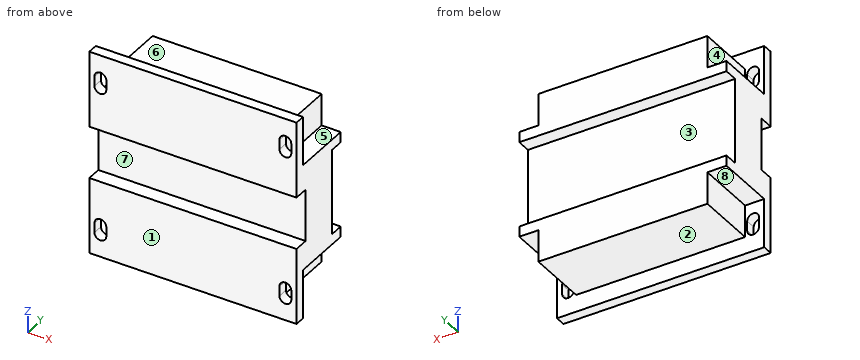
```python
from build123d import *

# Parameters (mm, degrees)
SKETCH1_W           = 75.692
SKETCH1_H           = 62.23
BOSS_EXTRUDE1_DEPTH = 25.908
SKETCH2_W           = 75.692
SKETCH2_H           = 31.242
CUT_EXTRUDE1_DEPTH  = 5.08
SKETCH4_W           = 6.985
SKETCH4_H           = 11.684
CUT_EXTRUDE4_DEPTH  = 22.098
SKETCH3_W           = 75.692
SKETCH3_H           = 19.05
CUT_EXTRUDE5_DEPTH  = 5.334
SKETCH8_W           = 75.692
SKETCH8_H           = 3.81
BOSS_EXTRUDE2_DEPTH = 6.223
SKETCH9_W           = 75.692
SKETCH9_H           = 3.81
BOSS_EXTRUDE3_DEPTH = 6.223
CUT_EXTRUDE6_REACH  = 84.92


with BuildPart() as part:
    # Sketch1 → Boss-Extrude1 (new body)
    with BuildSketch(Plane(origin=(0, 0, 0), x_dir=(1, 0, 0), z_dir=(0, 1, 0))):
        with Locations((-20.973907218, -15.051745981)):
            Rectangle(SKETCH1_W, SKETCH1_H)
    extrude(amount=BOSS_EXTRUDE1_DEPTH)

    # Sketch2 → Cut-Extrude1 (cut)
    with BuildSketch(Plane(origin=(0, 25.908, 0), x_dir=(1, 0, 0), z_dir=(0, 1, 0))):
        with Locations((-20.973907218, -15.051745981)):
            Rectangle(SKETCH2_W, SKETCH2_H)
    extrude(amount=-CUT_EXTRUDE1_DEPTH, mode=Mode.SUBTRACT)

    # Sketch4 → Cut-Extrude4 (cut)
    with BuildSketch(Plane(origin=(0, 25.908, 0), x_dir=(1, 0, 0), z_dir=(0, 1, 0))):
        with Locations((13.379592782, -40.324745981)):
            Rectangle(SKETCH4_W, SKETCH4_H)
        with Locations((-55.327407218, -40.324745981)):
            Rectangle(SKETCH4_W, SKETCH4_H)
        with Locations((-55.327407218, 10.221254019)):
            Rectangle(SKETCH4_W, SKETCH4_H)
        with Locations((13.379592782, 10.221254019)):
            Rectangle(SKETCH4_W, SKETCH4_H)
    extrude(amount=-CUT_EXTRUDE4_DEPTH, mode=Mode.SUBTRACT)

    # Sketch3 → Cut-Extrude5 (cut)
    with BuildSketch(Plane.XZ):
        with Locations((-20.973907218, 15.051745981)):
            Rectangle(SKETCH3_W, SKETCH3_H)
    extrude(amount=-CUT_EXTRUDE5_DEPTH, mode=Mode.SUBTRACT)

    # Sketch8 → Boss-Extrude2 (add)
    with BuildSketch(Plane.XY.offset(46.166745981)):
        with Locations((-20.973907218, 1.905)):
            Rectangle(SKETCH8_W, SKETCH8_H)
    extrude(amount=BOSS_EXTRUDE2_DEPTH)

    # Sketch9 → Boss-Extrude3 (add)
    with BuildSketch(Plane(origin=(0, 0, -16.063254019), x_dir=(-1, 0, 0), z_dir=(0, 0, -1))):
        with Locations((20.973907218, 1.905)):
            Rectangle(SKETCH9_W, SKETCH9_H)
    extrude(amount=BOSS_EXTRUDE3_DEPTH)

    # Sketch7 → Cut-Extrude6 (cut, up to next)
    with BuildSketch(Plane.XZ, mode=Mode.PRIVATE) as cut_extrude6_sk1:
        with BuildLine():
            Line((-56.914907218, 43.880745981), (-56.914907218, 40.324745981))
            ThreePointArc((-56.914907218, 40.324745981), (-54.755907218, 38.165745981), (-52.596907218, 40.324745981))
            Line((-52.596907218, 40.324745981), (-52.596907218, 43.880745981))
            ThreePointArc((-52.596907218, 43.880745981), (-54.755907218, 46.039745981), (-56.914907218, 43.880745981))
        make_face()
    cut_extrude6_tool1 = extrude(cut_extrude6_sk1.sketch, amount=-CUT_EXTRUDE6_REACH, mode=Mode.PRIVATE) & part.part
    # Sketch7 → Cut-Extrude6 (cut, up to next)
    with BuildSketch(Plane.XZ, mode=Mode.PRIVATE) as cut_extrude6_sk2:
        with BuildLine():
            Line((10.649092782, 43.880745981), (10.649092782, 40.324745981))
            ThreePointArc((10.649092782, 40.324745981), (12.808092782, 38.165745981), (14.967092782, 40.324745981))
            Line((14.967092782, 40.324745981), (14.967092782, 43.880745981))
            ThreePointArc((14.967092782, 43.880745981), (12.808092782, 46.039745981), (10.649092782, 43.880745981))
        make_face()
    cut_extrude6_tool2 = extrude(cut_extrude6_sk2.sketch, amount=-CUT_EXTRUDE6_REACH, mode=Mode.PRIVATE) & part.part
    # Sketch7 → Cut-Extrude6 (cut, up to next)
    with BuildSketch(Plane.XZ, mode=Mode.PRIVATE) as cut_extrude6_sk3:
        with BuildLine():
            Line((10.649092782, -10.475254019), (10.649092782, -14.031254019))
            ThreePointArc((10.649092782, -14.031254019), (12.808092782, -16.190254019), (14.967092782, -14.031254019))
            Line((14.967092782, -14.031254019), (14.967092782, -10.475254019))
            ThreePointArc((14.967092782, -10.475254019), (12.808092782, -8.316254019), (10.649092782, -10.475254019))
        make_face()
    cut_extrude6_tool3 = extrude(cut_extrude6_sk3.sketch, amount=-CUT_EXTRUDE6_REACH, mode=Mode.PRIVATE) & part.part
    # Sketch7 → Cut-Extrude6 (cut, up to next)
    with BuildSketch(Plane.XZ, mode=Mode.PRIVATE) as cut_extrude6_sk4:
        with BuildLine():
            Line((-56.914907218, -10.475254019), (-56.914907218, -14.031254019))
            ThreePointArc((-56.914907218, -14.031254019), (-54.755907218, -16.190254019), (-52.596907218, -14.031254019))
            Line((-52.596907218, -14.031254019), (-52.596907218, -10.475254019))
            ThreePointArc((-52.596907218, -10.475254019), (-54.755907218, -8.316254019), (-56.914907218, -10.475254019))
        make_face()
    cut_extrude6_tool4 = extrude(cut_extrude6_sk4.sketch, amount=-CUT_EXTRUDE6_REACH, mode=Mode.PRIVATE) & part.part
    add(cut_extrude6_tool1.solids().sort_by_distance((-54.755907, 0, 42.102746))[0], mode=Mode.SUBTRACT)
    add(cut_extrude6_tool2.solids().sort_by_distance((12.808093, 0, 42.102746))[0], mode=Mode.SUBTRACT)
    add(cut_extrude6_tool3.solids().sort_by_distance((12.808093, 0, -12.253254))[0], mode=Mode.SUBTRACT)
    add(cut_extrude6_tool4.solids().sort_by_distance((-54.755907, 0, -12.253254))[0], mode=Mode.SUBTRACT)


solid = part.part
```
Geometry check sheet. Reference: the model listing, model coordinates, mm. Face numbers are marked on the shaded views. A direction names the side the tool comes from. Round coordinates to 2 decimals unless told otherwise and drop trailing zeros. Loops run counter-clockwise (first coordinate to the right, second up) from the corner with the lowest first, then second, coordinate; pieces in that order, holes last. Notation, with made-up numbers: (-7, 27.5) - (5, 27.5) arc R14 ccw to (5, 47.5) - close; hole circle Ø11 at (88, 22.25). An arc over 180 degrees is marked (long way). Write item = value, one per line. Start each with the question number.
1. Section check D-D on z = 14.5. Enter the section's corners in (x, y).
2. Thickness scan on line 1 (Z direction, x = -34, y = 24.5); line 2 (Z direction, x = 6, y = 5); line 3 (Y direction, x = -5, z = 28). Record the ranges inside material, lowest first.
3. Set-up check for the marked faces 4, 5, 6, 7 and 8: record each of +Z, -Z, +X, -X, +Y, -Y from which the full face is reachable in a straight line by a thin tool's end or side.
4. Section check B-B on y = 7.5. Enter the section's corners in (x, z), then the cut area to 3 significant figures.
5. Section check A-A on z = -13. Enter the section's corners in (x, y).
6. Mould release check, pull along Z, two halves, no side actions. Record for the marked faces 1, 2 and 3: released by +Z, released by -Z, zero draft, split by the parting line, or undercut.
7. Depth check by flat-ended pin: pin 1 (5.5 mm diameter, centred on x = -12, y = 22.5, fed in from +Z); pin 2 (9.5 mm diameter, centred on x = -37, z = 10.5, fed in from +Y); pin 3 (2 mm diameter, centred on y = 6.5, z = 41, fed in from +X); pin 4 (12 mm diameter, centred on y = 8, z = -14.5, fed in from +X). Enter the tip coordinate at first touch or a pass-through.
8. Section check C-C on x = -15. Enter the section's corners in (y, z).
Working result:
q1.outline = (-58.82, 5.33) - (16.87, 5.33) - (16.87, 20.83) - (-58.82, 20.83) - close
q2.line_1 = -16.06 to -0.57, 30.67 to 46.17
q2.line_2 = -16.06 to 5.53, 24.58 to 46.17
q2.line_3 = 0 to 20.83
q3.face_4 = +Z, -X, +Y
q3.face_5 = +Z, +X, +Y
q3.face_6 = +Z, +X, -X, +Y
q3.face_7 = +X, -X, -Y
q3.face_8 = -Z, -X, +Y
q4.outline = (-58.82, -4.38) - (-51.83, -4.38) - (-51.83, -16.06) - (9.89, -16.06) - (9.89, -4.38) - (16.87, -4.38) - (16.87, 34.48) - (9.89, 34.48) - (9.89, 46.17) - (-51.83, 46.17) - (-51.83, 34.48) - (-58.82, 34.48) - close
q4.area = 4,380 mm^2
q5.outline = (-58.82, 0) - (-56.91, 0) - (-56.91, 3.81) - (-58.82, 3.81) - close; (-52.6, 0) - (10.65, 0) - (10.65, 3.81) - (9.89, 3.81) - (9.89, 25.91) - (-51.83, 25.91) - (-51.83, 3.81) - (-52.6, 3.81) - close; (14.97, 0) - (16.87, 0) - (16.87, 3.81) - (14.97, 3.81) - close
q6.face_1 = zero draft
q6.face_2 = released by -Z
q6.face_3 = undercut
q7.pin_1 = 46.17
q7.pin_2 = 20.83
q7.pin_3 = 9.89
q7.pin_4 = 16.87
q8.outline = (0, -22.29) - (3.81, -22.29) - (3.81, -16.06) - (25.91, -16.06) - (25.91, -0.57) - (20.83, -0.57) - (20.83, 30.67) - (25.91, 30.67) - (25.91, 46.17) - (3.81, 46.17) - (3.81, 52.39) - (0, 52.39) - (0, 24.58) - (5.33, 24.58) - (5.33, 5.53) - (0, 5.53) - close
